For this review, take the finished solid that the model builds, in its own axes (mm). Round coordinates to 2 decimals unless told otherwise and drop trailing zeros. Order: outer loops, then holes, each group sorted by start corner. A loop starts at its lowest first (then second) coordinate and runs counter-clockwise, first axis right, second up. Notation, with made-up numbers: (-1, -29) -> (49, -29) arc R24 ccw to (49, 0) -> close; hole circle Ø1 at (-31.75, 73). An arc over 180 degrees is marked (long way). Answer in a Markdown table with one row per item.
```python
from build123d import *

# Parameters (mm, degrees)
ESQUISSE1_R                  = 3
BOSS_EXTRU_1_DEPTH           = 2
CONG_1_R                     = 18
CONG_2_R                     = 20
ENL_V_MAT_EXTRU_2_DEPTH      = 195.530962239
ENL_V_MAT_EXTRU_2_DEPTH_BACK = 10
ESQUISSE2_W                  = 356.718168982
ESQUISSE2_H                  = 96.805953854
D_GAGEMENT_M31_D             = 3.4


with BuildPart() as part:
    # Esquisse1 → Boss.-Extru.1 (new body)
    with BuildSketch(Plane.XY):
        Polygon((-244.958991582, 40), (-110, 40), (110, 40), (244.958991582, 40), (112.479495791, -30), (-112.479495791, -30), align=None)
        with Locations((-175, 20)):
            Circle(ESQUISSE1_R, mode=Mode.SUBTRACT)
        with Locations((-110, -20)):
            Circle(ESQUISSE1_R, mode=Mode.SUBTRACT)
        with Locations((110, -20)):
            Circle(ESQUISSE1_R, mode=Mode.SUBTRACT)
        with Locations((175, 20)):
            Circle(ESQUISSE1_R, mode=Mode.SUBTRACT)
        with Locations((0, -20)):
            Circle(ESQUISSE1_R, mode=Mode.SUBTRACT)
        with Locations((-58.333333333, 20)):
            Circle(ESQUISSE1_R, mode=Mode.SUBTRACT)
        with Locations((58.333333333, 20)):
            Circle(ESQUISSE1_R, mode=Mode.SUBTRACT)
    extrude(amount=BOSS_EXTRU_1_DEPTH)

    # Congé1
    cong_1_edges = [part.edges().sort_by_distance(p)[0] for p in [
        (-244.958991582, 40, 1),
        (244.958991582, 40, 1),
    ]]
    fillet(cong_1_edges, radius=CONG_1_R)

    # Congé2
    cong_2_edges = [part.edges().sort_by_distance(p)[0] for p in [
        (112.479495791, -30, 1),
        (-112.479495791, -30, 1),
    ]]
    fillet(cong_2_edges, radius=CONG_2_R)

    # Esquisse2 → Enlèv. mat.-Extru.2 (cut, two sides: drawn at the far end of the back side and taken through both)
    with BuildSketch(Plane.XY.offset(-ENL_V_MAT_EXTRU_2_DEPTH_BACK)):
        with Locations((23.359084491, 12.745190259)):
            Rectangle(ESQUISSE2_W, ESQUISSE2_H)
    extrude(amount=ENL_V_MAT_EXTRU_2_DEPTH + ENL_V_MAT_EXTRU_2_DEPTH_BACK, mode=Mode.SUBTRACT)

    # Dégagement M31 (through all)
    with Locations(Plane(origin=(0, 0, 0), x_dir=(-1, 0, 0), z_dir=(0, 0, -1))):
        with Locations((160, 33.228756555), (160, 6.771243445)):
            Hole(D_GAGEMENT_M31_D / 2)


solid = part.part
```
Q1. Clearance check with flat-ended pins moving along their axes: pin 1 Ø3 at (x, y) = (-160, 6.77) entering from -Z; pin 2 Ø7 at (x, y) = (-175, 20) entering from +Z. State where each tip first meets the part, or that it passes through.
Answer key:
| item | result |
|---|---|
| pin 1 | passes through |
| pin 2 | stops at z = 2 |
Q2. Take a section at D-D, the plane x = -159. Write out the cut boundary in (y, z), then the cut area to 3 significant figures.
Answer key:
| item | result |
|---|---|
| outline | (-5.42, 0) -> (5.4, 0) -> (5.4, 2) -> (-5.42, 2) -> close; (8.15, 0) -> (31.85, 0) -> (31.85, 2) -> (8.15, 2) -> close; (34.6, 0) -> (40, 0) -> (40, 2) -> (34.6, 2) -> close |
| area | 79.8 mm^2 |
Q3. Take a section at B-B, the plane y = 20. Write out the cut boundary in (x, z), then the cut area to 3 significant figures.
Answer key:
| item | result |
|---|---|
| outline | (-190.25, 0) -> (-178, 0) -> (-178, 2) -> (-190.25, 2) -> close; (-172, 0) -> (-155, 0) -> (-155, 2) -> (-172, 2) -> close |
| area | 58.5 mm^2 |
Q4. The part is to be moulded in two halves that separate along Y. For faces 1 (the face through (-167.706, -0.819, 0.986)), 2 (the face through (-172.14, 20.9, 0.99)), 3 (the face through (-169, 22, 0)), say which applies: +Y half, -Y half, draft (parallel to the pull), parting line (faces both ways), or undercut.
Answer key:
| item | result |
|---|---|
| face 1 | -Y half |
| face 2 | undercut |
| face 3 | draft |
Q5. Take a section at C-C, the plane z = 0.7. Write out the cut boundary in (x, y), then the cut area to 3 significant figures.
Answer key:
| item | result |
|---|---|
| outline | (-180.77, 6.09) -> (-155, -7.53) -> (-155, 40) -> (-172.36, 40) arc R18 ccw to start; hole circle Ø6 at (-175, 20); hole circle Ø3.4 at (-160, 6.77); hole circle Ø3.4 at (-160, 33.23) |
| area | 1,220 mm^2 |
Q6. Take a section at A-A, the plane x = -175. Write out the cut boundary in (y, z).
Answer key:
| item | result |
|---|---|
| outline | (3.03, 0) -> (17, 0) -> (17, 2) -> (3.03, 2) -> close; (23, 0) -> (39.81, 0) -> (39.81, 2) -> (23, 2) -> close |
Q7. To check wall thickness, follow probe 1 along Y at (x, z) = (-160, 1.25); probe 2 along Y at (x, z) = (-172.5, 0.85); probe 3 along Y at (x, z) = (-175, 1.3). State the ranges of each line that lie inside material, in increasing order.
Answer key:
| item | result |
|---|---|
| probe 1 | y = -4.89 to 5.07, 8.47 to 31.53, 34.93 to 40 |
| probe 2 | y = 1.71 to 18.34, 21.66 to 40 |
| probe 3 | y = 3.03 to 17, 23 to 39.81 |
